Source: CAD feature listing. Evaluate the final solid. Frame: model axes, mm. Round coordinates to 2 decimals unless told otherwise and drop trailing zeros. Order: outer loops, then holes, each group sorted by start corner. A loop starts at its lowest first (then second) coordinate and runs counter-clockwise, first axis right, second up. Notation, with made-up numbers: (17.5, -26.75) - (43.5, -26.75) arc R21 ccw to (43.5, -19.75) - close; hole circle Ø7 at (-8, -6). An arc over 180 degrees is marked (long way). Return JSON: item names as keys, results as strings. Group by question number.
1) Ray query, line 1 (X direction, y = -2.4, z = -7.75); line 2 (X direction, y = -2.75, z = -5); line 3 (Z direction, x = 7.25, y = -1.7). Return the intervals inside material, ascending. Write a range as from..to.
2) Section C-C, the plane y = -2.5. Return loops of the section in (x, z).
3) Section B-B, the plane z = -1. Return loops of the section in (x, y).
4) Section A-A, the plane x = 8.5. Return loops of the section in (y, z).
Autodesk Inventor part; units mm, degrees
ref_plane "YZ Plane" through (0, 0, 0) normal (1, 0, 0) x (0, 1, 0)
ref_plane "XZ Plane" through (0, 0, 0) normal (0, 1, 0) x (-1, 0, 0)
ref_plane "XY Plane" through (0, 0, 0) normal (0, 0, 1) x (1, 0, 0)
sketch "Sketch1" plane through (0, 0, 0) normal (0, 1, 0) x (-1, 0, 0)
  line L0 (0, 0) -> (-9.9, 0)
  line L1 (0, 0) -> (0, -10.3)
  line L2 (0, -10.3) -> (-9.9, -10.3)
  line L3 (-9.9, -10.3) -> (-9.9, 0)
  line L4 (-9.9, -10.3) -> (-9.4, -10.3)
  line L5 (-9.4, -10.3) -> (-9.4, 0)
  line L6 (0, -10.3) -> (-0.5, -10.3)
  line L7 (-0.5, -10.3) -> (-0.5, 0)
  line L8 (-0.5, 0.85) -> (-9.9, 0.85)
  line L9 (-9.9, 0.85) -> (-9.9, 0)
  line L10 (0, 0) -> (0, 0.85)
  line L11 (0, 0.85) -> (-0.5, 0.85)
  line L12 (0, -10.3) -> (0, -11.15)
  line L13 (0, -11.15) -> (-9.9, -11.15)
  line L14 (-9.9, -11.15) -> (-9.9, -10.3)
  line L15 (-9.9, -11.15) -> (-19.8, -11.15)
  line L16 (-19.8, -11.15) -> (-19.8, -10.3)
  line L17 (-19.8, -10.3) -> (-19.8, 0)
  line L18 (-19.3, -10.3) -> (-19.3, 0)
  line L19 (-9.9, -10.3) -> (-19.8, -10.3)
  line L20 (-10.4, -10.3) -> (-10.4, 0)
  line L21 (-9.9, 0) -> (-9.9, -10.3)
  line L22 (-9.9, 0) -> (-9.9, 0.85)
  line L23 (-9.9, 0.85) -> (-10.4, 0.85)
  line L24 (-10.4, 0.85) -> (-19.8, 0.85)
  line L25 (-9.9, 0) -> (-19.8, 0)
  line L26 (-19.8, 0.85) -> (-19.8, 0)
  line L27 (-19.8, -11.15) -> (-29.7, -11.15)
  line L28 (-29.7, -11.15) -> (-29.7, -10.3)
  line L29 (-29.7, -10.3) -> (-29.7, 0)
  line L30 (-29.2, -10.3) -> (-29.2, 0)
  line L31 (-19.8, -10.3) -> (-29.7, -10.3)
  line L32 (-20.3, -10.3) -> (-20.3, 0)
  line L33 (-19.8, 0) -> (-19.8, -10.3)
  line L34 (-19.8, 0) -> (-19.8, 0.85)
  line L35 (-19.8, 0.85) -> (-20.3, 0.85)
  line L36 (-20.3, 0.85) -> (-29.7, 0.85)
  line L37 (-19.8, 0) -> (-29.7, 0)
  line L38 (-29.7, 0.85) -> (-29.7, 0)
  line L39 (-29.7, -11.15) -> (-39.6, -11.15)
  line L40 (-39.6, -11.15) -> (-39.6, -10.3)
  line L41 (-39.6, -10.3) -> (-39.6, 0)
  line L42 (-39.1, -10.3) -> (-39.1, 0)
  line L43 (-29.7, -10.3) -> (-39.6, -10.3)
  line L44 (-30.2, -10.3) -> (-30.2, 0)
  line L45 (-29.7, 0) -> (-29.7, -10.3)
  line L46 (-29.7, 0) -> (-29.7, 0.85)
  line L47 (-29.7, 0.85) -> (-30.2, 0.85)
  line L48 (-30.2, 0.85) -> (-39.6, 0.85)
  line L49 (-29.7, 0) -> (-39.6, 0)
  line L50 (-39.6, 0.85) -> (-39.6, 0)
  line L51 (-39.6, -11.15) -> (-49.5, -11.15)
  line L52 (-49.5, -11.15) -> (-49.5, -10.3)
  line L53 (-49.5, -10.3) -> (-49.5, 0)
  line L54 (-49, -10.3) -> (-49, 0)
  line L55 (-39.6, -10.3) -> (-49.5, -10.3)
  line L56 (-40.1, -10.3) -> (-40.1, 0)
  line L57 (-39.6, 0) -> (-39.6, -10.3)
  line L58 (-39.6, 0) -> (-39.6, 0.85)
  line L59 (-39.6, 0.85) -> (-40.1, 0.85)
  line L60 (-40.1, 0.85) -> (-49.5, 0.85)
  line L61 (-39.6, 0) -> (-49.5, 0)
  line L62 (-49.5, 0.85) -> (-49.5, 0)
  line L63 (-49.5, -11.15) -> (-59.4, -11.15)
  line L64 (-59.4, -11.15) -> (-59.4, -10.3)
  line L65 (-59.4, -10.3) -> (-59.4, 0)
  line L66 (-58.9, -10.3) -> (-58.9, 0)
  line L67 (-49.5, -10.3) -> (-59.4, -10.3)
  line L68 (-50, -10.3) -> (-50, 0)
  line L69 (-49.5, 0) -> (-49.5, -10.3)
  line L70 (-49.5, 0) -> (-49.5, 0.85)
  line L71 (-49.5, 0.85) -> (-50, 0.85)
  line L72 (-50, 0.85) -> (-59.4, 0.85)
  line L73 (-49.5, 0) -> (-59.4, 0)
  line L74 (-59.4, 0.85) -> (-59.4, 0)
  line L75 (-59.4, -11.15) -> (-69.3, -11.15)
  line L76 (-69.3, -11.15) -> (-69.3, -10.3)
  line L77 (-69.3, -10.3) -> (-69.3, 0)
  line L78 (-68.8, -10.3) -> (-68.8, 0)
  line L79 (-59.4, -10.3) -> (-69.3, -10.3)
  line L80 (-59.9, -10.3) -> (-59.9, 0)
  line L81 (-59.4, 0) -> (-59.4, -10.3)
  line L82 (-59.4, 0) -> (-59.4, 0.85)
  line L83 (-59.4, 0.85) -> (-59.9, 0.85)
  line L84 (-59.9, 0.85) -> (-69.3, 0.85)
  line L85 (-59.4, 0) -> (-69.3, 0)
  line L86 (-69.3, 0.85) -> (-69.3, 0)
  line L87 (-69.3, -11.15) -> (-79.2, -11.15)
  line L88 (-79.2, -11.15) -> (-79.2, -10.3)
  line L89 (-79.2, -10.3) -> (-79.2, 0)
  line L90 (-78.7, -10.3) -> (-78.7, 0)
  line L91 (-69.3, -10.3) -> (-79.2, -10.3)
  line L92 (-69.8, -10.3) -> (-69.8, 0)
  line L93 (-69.3, 0) -> (-69.3, -10.3)
  line L94 (-69.3, 0) -> (-69.3, 0.85)
  line L95 (-69.3, 0.85) -> (-69.8, 0.85)
  line L96 (-69.8, 0.85) -> (-79.2, 0.85)
  line L97 (-69.3, 0) -> (-79.2, 0)
  line L98 (-79.2, 0.85) -> (-79.2, 0)
  line L99 (-79.2, -11.15) -> (-89.1, -11.15)
  line L100 (-89.1, -11.15) -> (-89.1, -10.3)
  line L101 (-89.1, -10.3) -> (-89.1, 0)
  line L102 (-88.6, -10.3) -> (-88.6, 0)
  line L103 (-79.2, -10.3) -> (-89.1, -10.3)
  line L104 (-79.7, -10.3) -> (-79.7, 0)
  line L105 (-79.2, 0) -> (-79.2, -10.3)
  line L106 (-79.2, 0) -> (-79.2, 0.85)
  line L107 (-79.2, 0.85) -> (-79.7, 0.85)
  line L108 (-79.7, 0.85) -> (-89.1, 0.85)
  line L109 (-79.2, 0) -> (-89.1, 0)
  line L110 (-89.1, 0.85) -> (-89.1, 0)
  line L111 (-89.1, -11.15) -> (-99, -11.15)
  line L112 (-99, -11.15) -> (-99, -10.3)
  line L113 (-99, -10.3) -> (-99, 0)
  line L114 (-98.5, -10.3) -> (-98.5, 0)
  line L115 (-89.1, -10.3) -> (-99, -10.3)
  line L116 (-89.6, -10.3) -> (-89.6, 0)
  line L117 (-89.1, 0) -> (-89.1, -10.3)
  line L118 (-89.1, 0) -> (-89.1, 0.85)
  line L119 (-89.1, 0.85) -> (-89.6, 0.85)
  line L120 (-89.6, 0.85) -> (-99, 0.85)
  line L121 (-89.1, 0) -> (-99, 0)
  line L122 (-99, 0.85) -> (-99, 0)
  line L123 (0, -11.15) -> (0, 0.85)
  line L124 (0, -11.15) -> (0, -12.65)
  line L125 (0, -12.65) -> (1.5, -12.65)
  line L126 (-99, 0.85) -> (-100.5, 0.85)
  line L127 (-100.5, 0.85) -> (-100.5, 2.35)
  line L128 (1.5, -12.65) -> (-100.5, -12.65)
  line L129 (-100.5, -12.65) -> (-100.5, 2.35)
  line L130 (-100.5, 2.35) -> (1.5, 2.35)
  line L131 (1.5, 2.35) -> (1.5, -12.65)
  line L132 (0, -11.15) -> (1.5, -11.15)
  line L133 (0, 0.85) -> (1.5, 0.85)
  line L134 (0, -11.15) -> (-2, -11.15)
  line L135 (-2, -11.15) -> (-2, 0.85)
  point P0 (-2, -10.3)
  point P1 (-2, 0)
  dimension "d0" = 9.9
  dimension "d1" = 10.3
  dimension "d2" = 0.5
  dimension "d3" = 0.5
  dimension "d6" = 0.85
  dimension "d7" = 0.85
  dimension "d10" = 9.9
  dimension "d15" = 1.5
  dimension "d16" = 1.5
  dimension "d19" = 1.5
  dimension "d20" = 2
extrude "Extrusion3" add sketch "Sketch1" against normal blind 3 contours L7 L2 L135 L0 | L135 L2 L5 L0
chamfer "Chamfer1" distance 1.5 angle 45 4 edges at (4.95, -3, 0) (9.4, -3, -5.15) (0.5, -3, -5.15) (4.95, -3, -10.3)
extrude "Extrusion4" add sketch "Sketch1" along normal blind 1.5 contours L7 L2 L135 L0 | L135 L2 L5 L0
properties part number "10x led strip diffuser"
Geometry check:
{
 "1": {"line 1": "1.4..8.5", "line 2": "1.75..8.15", "line 3": "-10.1..-0.2"},
 "2": {"outline": "(1.5, -9.3) - (8.4, -9.3) - (8.4, -1) - (1.5, -1) - close"},
 "3": {"outline": "(0.5, -1.5) - (1.5, -2.5) - (8.4, -2.5) - (9.4, -1.5) - (9.4, 1.5) - (0.5, 1.5) - close"},
 "4": {"outline": "(-2.4, -9.4) - (-1.5, -10.3) - (1.5, -10.3) - (1.5, 0) - (-1.5, 0) - (-2.4, -0.9) - close"}
}
